Autodesk Inventor part; units mm, degrees
ref_plane "YZ Plane" through (0, 0, 0) normal (1, 0, 0) x (0, 1, 0)
ref_plane "XZ Plane" through (0, 0, 0) normal (0, 1, 0) x (-1, 0, 0)
ref_plane "XY Plane" through (0, 0, 0) normal (0, 0, 1) x (1, 0, 0)
sketch "Sketch1" plane through (0, 0, 0) normal (0, 0, 1) x (1, 0, 0)
  line L0 (-178.79, -80) -> (6.21, -80)
  line L1 (6.21, 80) -> (-178.79, 80)
  line L2 (-183.79, 75) -> (-183.79, -75)
  circle A0 centre (41, 41) radius 2
  circle A1 centre (41, -41) radius 2
  circle A2 centre (-41, -41) radius 2
  circle A3 centre (-41, 41) radius 2
  line L3 (86.21, 0) -> (86.21, 0)
  arc A4 (6.21, -80) -> (86.21, 0) centre (6.21, 0) ccw
  arc A5 (86.21, 0) -> (6.21, 80) centre (6.21, 0) ccw
  circle A6 centre (81.21, 0) radius 1.5
  circle A7 centre (59.243, -53.033) radius 1.5
  circle A8 centre (6.21, -75) radius 1.5
  circle A9 centre (-48.79, -75) radius 1.5
  circle A10 centre (-103.79, -75) radius 1.5
  circle A11 centre (-178.79, -75) radius 1.5
  circle A12 centre (-178.79, 0) radius 1.5
  circle A13 centre (-178.79, 75) radius 1.5
  circle A14 centre (-103.79, 75) radius 1.5
  circle A15 centre (-48.79, 75) radius 1.5
  circle A16 centre (6.21, 75) radius 1.5
  circle A17 centre (59.243, 53.033) radius 1.5
  circle A18 centre (12, 65) radius 1.1
  circle A19 centre (12, 58) radius 1.1
  arc A20 (-117.0042, -28.5) -> (-117.0042, -25.5) centre (-117.0042, -27) ccw
  line L4 (-117.0042, -28.5) -> (-121.0042, -28.5)
  line L5 (-117.0042, -25.5) -> (-121.0042, -25.5)
  arc A21 (-121.0042, -25.5) -> (-121.0042, -28.5) centre (-121.0042, -27) ccw
  arc A22 (-121.0042, -56.5) -> (-121.0042, -59.5) centre (-121.0042, -58) ccw
  line L6 (-117.0042, -59.5) -> (-121.0042, -59.5)
  line L7 (-117.0042, -56.5) -> (-121.0042, -56.5)
  arc A23 (-117.0042, -59.5) -> (-117.0042, -56.5) centre (-117.0042, -58) ccw
  arc A24 (-105.5042, -31.5) -> (-105.5042, -53.5) centre (-105.5042, -42.5) ccw
  arc A25 (-101.5042, -53.5) -> (-101.5042, -31.5) centre (-101.5042, -42.5) ccw
  line L8 (-101.5042, -31.5) -> (-105.5042, -31.5)
  line L9 (-101.5042, -53.5) -> (-105.5042, -53.5)
  arc A26 (-86.0042, -28.5) -> (-86.0042, -25.5) centre (-86.0042, -27) ccw
  line L10 (-86.0042, -28.5) -> (-90.0042, -28.5)
  line L11 (-86.0042, -25.5) -> (-90.0042, -25.5)
  arc A27 (-90.0042, -25.5) -> (-90.0042, -28.5) centre (-90.0042, -27) ccw
  arc A28 (-86.0042, -59.5) -> (-86.0042, -56.5) centre (-86.0042, -58) ccw
  line L12 (-86.0042, -59.5) -> (-90.0042, -59.5)
  line L13 (-86.0042, -56.5) -> (-90.0042, -56.5)
  arc A29 (-90.0042, -56.5) -> (-90.0042, -59.5) centre (-90.0042, -58) ccw
  arc A30 (-183.79, -75) -> (-178.79, -80) centre (-178.79, -75) ccw
  arc A31 (-178.79, 80) -> (-183.79, 75) centre (-178.79, 75) ccw
  point P0 (0, 0)
  point P1 (-183.79, -80)
  point P2 (-183.79, 80)
  point P3 (0, 0)
  point P4 (86.21, 0)
  point P5 (-103.5042, -42.5)
  point P6 (-103.5042, -42.5)
  point P7 (86.21, 0)
  point P8 (-119.0042, -58)
  point P9 (-103.5042, -42.5)
  point P10 (-103.5042, -53.5)
  point P11 (-119.0042, -25.5)
  point P12 (-119.0042, -28.5)
  dimension "d5" = 4
  dimension "d10" = 80
  dimension "d12" = 3
  dimension "d15" = 3
  dimension "d17" = 3
  dimension "d21" = 3
  dimension "d22" = 3
  dimension "d23" = 3
  dimension "d24" = 3
  dimension "d39" = 3
  dimension "d40" = 1.5
  dimension "d41" = 22
  dimension "d42" = 11
  dimension "d44" = 80
  dimension "d45" = 6.21
  dimension "d46" = 183.79
  dimension "d51" = 3
  dimension "d56" = 5
  dimension "d57" = 5
  dimension "d58" = 5
  dimension "d59" = 5
  dimension "d60" = 3
  dimension "d61" = 3
  dimension "d62" = 5
  dimension "d63" = 80
  dimension "d64" = 5
  dimension "d65" = 3
  dimension "d66" = 4
  dimension "d67" = 135
  dimension "d68" = 41
  dimension "d91" = 3
  dimension "d92" = 1.5
  dimension "d96" = 3
  dimension "d97" = 1.5
  dimension "d99" = 41
  dimension "d100" = 82
  dimension "d101" = 4
  dimension "d102" = 4
  dimension "d103" = 82
  dimension "d104" = 7
  dimension "d105" = 3
  dimension "d106" = 6.21
  dimension "d107" = 58
  dimension "d108" = 12
  dimension "d109" = 2.2
  dimension "d110" = 2.2
  dimension "d113" = 37.5
  dimension "d114" = 80.2858
  dimension "d115" = 2
  dimension "d116" = 2
  dimension "d117" = 80.2858
  dimension "d118" = 37.5
  dimension "d119" = 11
  dimension "d120" = 4
  dimension "d124" = 4
  dimension "d125" = 3
  dimension "d126" = 15.5
  dimension "d127" = 15.5
  dimension "d128" = 1.5
  dimension "d129" = 13.5
  dimension "d130" = 2
  dimension "d131" = 2
  dimension "d132" = 1.5
  dimension "d133" = 1.5
extrude "Extrusion1" add sketch "Sketch1" along normal blind 4
equation "\"d15\" = d12"
equation "\"d17\" = d12"
equation "\"d21\" = d12"
equation "\"d22\" = d12"
equation "\"d23\" = d12"
equation "\"d24\" = d12"
equation "\"d39\" = d31"
equation "\"d40\" = 0.5 * d31"
equation "\"d41\" = d9"
equation "\"d42\" = 0.5 * d9"
equation "\"d91\" = d89"
equation "\"d92\" = 0.5 * d89"
equation "\"d96\" = d94"
equation "\"d97\" = 0.5 * d94"
properties part number "testbaseup"
Geometry check sheet. Reference: the model listing, model coordinates, mm. A direction names the side the tool comes from. Round coordinates to 2 decimals unless told otherwise and drop trailing zeros. Loops run counter-clockwise (first coordinate to the right, second up) from the corner with the lowest first, then second, coordinate; pieces in that order, holes last. Notation, with made-up numbers: (-36, 5.25) -> (14, 5.25) arc R30 cw to (14, 28.25) -> close; hole circle Ø1 at (-33, 20.5). An arc over 180 degrees is marked (long way). Use a Markdown table: item, result.
(1) Mould release check, pull along X, two halves, no side actions. Record for faces 3 (the flat face through (-51, 1, 4)), 4 (the cylindrical face through (86.19, 1.76, 1.97)), 5 (the cylindrical face through (-90.507, -42.258, 1.972)): released by +X, released by -X, zero draft, split by the parting line, or undercut.
Calculated:
| item | result |
|---|---|
| face 3 | zero draft |
| face 4 | released by +X |
| face 5 | undercut |
(2) Set-up check for faces 1 (the cylindrical face through (-182.29, -78.57, 1.97)), 2 (the cylindrical face through (-116.5, -42.74, 1.97)): record each of +Z, -Z, +X, -X, +Y, -Y from which the full face is reachable in a straight line by a thin tool's end or side.
Calculated:
| item | result |
|---|---|
| face 1 | +Z, -Z, -X, -Y |
| face 2 | +Z, -Z |
(3) Scan lines: probe 1 along Y at (x, z) = (6.21, 2.6); probe 2 along Y at (x, z) = (-121, 0.7); probe 3 along X at (y, z) = (-2.5, 2.9). Record each from-to range of solid material in increasing order.
Calculated:
| item | result |
|---|---|
| probe 1 | -80 to -76.5, -73.5 to 73.5, 76.5 to 80 |
| probe 2 | -80 to -59.5, -56.5 to -28.5, -25.5 to 80 |
| probe 3 | -183.79 to 86.17 |
(4) Sectioned sample at A-A (y = 46). Enter the section's corners in (x, z), then the cut area to 3 significant figures.
Calculated:
| item | result |
|---|---|
| outline | (-183.79, 0) -> (71.66, 0) -> (71.66, 4) -> (-183.79, 4) -> close |
| area | 1,020 mm² |
(5) Go/stop test with flat-tipped pins: P1, Ø1, axis at y = -35.5, z = 0.5, coming from the +X side; P2, Ø3, axis at x = 41, y = -41, coming from the +Z side; P3, Ø2, axis at y = 45.5, z = 3, coming from the +X side. Record where each tip stops, or that it passes through.
Calculated:
| item | result |
|---|---|
| P1 | x = 78.15 |
| P2 | through |
| P3 | x = 72.69 |
(6) Sectioned sample at C-C (z = 2.65). Give the number of separate pieces and of enclosed holes in the cut face, then the cut area to 3 significant figures.
Calculated:
| item | result |
|---|---|
| separate pieces | 1 |
| enclosed holes | 23 |
| area | 39,800 mm² |
(7) Sectioned sample at B-B (x = 55). Enter the section's corners in (y, z).
Calculated:
| item | result |
|---|---|
| outline | (-63.4, 0) -> (63.4, 0) -> (63.4, 4) -> (-63.4, 4) -> close |
